Geometry check sheet. Reference: the model listing, model coordinates, mm. Face numbers are marked on the shaded views. Round coordinates to 2 decimals unless told otherwise and drop trailing zeros. Order: outer loops, then holes, each group sorted by start corner. A loop starts at its lowest first (then second) coordinate and runs counter-clockwise, first axis right, second up.
(1) Sectioned sample at C-C (z = -8). Record the boundary of the cut face in (x, y), plus the area to 3 significant figures.
(2) Release check for a two-part mould opening along X. For the marked faces 1, 2 and 3 record: +X half, -X half, draft (parallel to the pull), parting line (faces both ways), or undercut.
(3) Go/stop test with flat-tipped pins: pin 1 (8 mm diameter, centred on x = 11.5, y = -7.5, fed in from -Z); pin 2 (1.5 mm diameter, centred on x = -8, z = 2.5, fed in from +Y); pin 3 (1 mm diameter, centred on y = -1, z = 3.5, fed in from +X). Record where each tip stops, or that it passes through.
(4) Sectioned sample at D-D (z = 3). Record the boundary of the cut face in (x, y).
(5) Sectioned sample at A-A (x = 0). Record the boundary of the cut face in (y, z).
(6) Material ranges on line 1 along X through (y, z) = (0, 1.25); line 2 along X through (y, z) = (-8, 7.5); line 3 along Y through (x, z) = (-3, -4), recorded low to high.
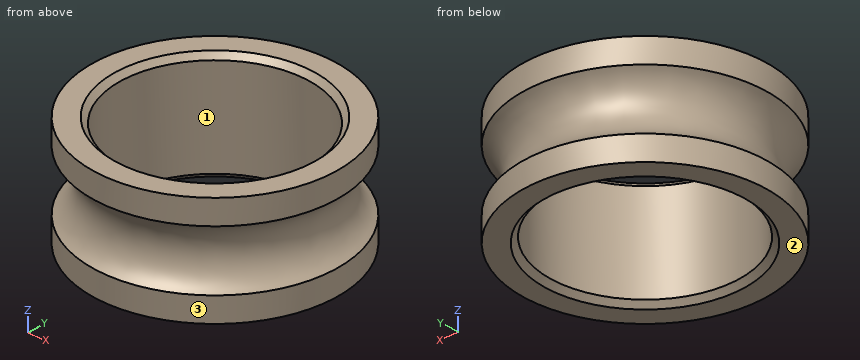
Solid Edge part; units mm, degrees
sketch "Sketch1" plane through (0, 0, 0) normal (0, -1, 0) x (1, 0, 0)
  line L0 (17.5, 10) -> (17.5, -10)
  line L1 (17.5, -10) -> (22.5, -10)
  line L2 (22.5, -10) -> (22.5, 10)
  line L3 (22.5, 10) -> (17.5, 10)
  dimension "D1" = 22.5
  dimension "D2" = 22.5
revolve "RevolvedProtrusion1" add sketch "Sketch1" angle 360 about axis through (0, 0, 54) along (0, 0, -1)
chamfer "Chamfer1" distance 1 angle 45 2 edges at (-17.5, 0, 10) (-17.5, 0, -10)
sketch "Sketch2" plane through (0, 0, 0) normal (0, -1, 0) x (1, 0, 0)
  circle A0 centre (26, 0) radius 6.5
revolve "RevolvedCutout1" cut sketch "Sketch2" angle 360 about axis through (0, 0, 54) along (0, 0, -1)
properties material "Polyethylene, low density"
Answer below:
1. outline: circle Ø45 at (0, 0); hole circle Ø35 at (0, 0)
1. area: 628 mm2
2. face 1: undercut
2. face 2: draft
2. face 3: parting line
3. pin 1: stops at z = -9.23
3. pin 2: stops at y = 18.83
3. pin 3: stops at x = 20.85
4. outline: circle Ø40.47 at (0, 0); hole circle Ø35 at (0, 0)
5. outline: (-22.5, -10) - (-18.5, -10) - (-17.5, -9) - (-17.5, 9) - (-18.5, 10) - (-22.5, 10) - (-22.5, 5.48) arc R6.5 cw to (-22.5, -5.48) - close; (17.5, -9) - (18.5, -10) - (22.5, -10) - (22.5, -5.48) arc R6.5 cw to (22.5, 5.48) - (22.5, 10) - (18.5, 10) - (17.5, 9) - close
6. line 1: x = -19.62 to -17.5, 17.5 to 19.62
6. line 2: x = -21.03 to -15.56, 15.56 to 21.03
6. line 3: y = -20.66 to -17.24, 17.24 to 20.66
